from build123d import *

# Parameters (mm, degrees)
SKETCH1_R           = 22.05
BOSS_EXTRUDE1_DEPTH = 8
CUT_EXTRUDE1_REACH  = 54.573
SKETCH2_R           = 4
CUT_EXTRUDE2_REACH  = 54.573
FILLET1_SIZE        = 1
BOSS_EXTRUDE2_START = 6
SKETCH4_W           = 14
SKETCH4_H           = 20
SKETCH4_R           = 4
BOSS_EXTRUDE2_DEPTH = 6
SKETCH6_W           = 12.1
SKETCH6_H           = 8.1
CUT_EXTRUDE3_DEPTH  = 2
SKETCH7_R           = 1.25
CUT_EXTRUDE4_DEPTH  = 8
FILLET2_R           = 1


with BuildPart() as part:
    # Sketch1 → Boss-Extrude1 (new body)
    with BuildSketch(Plane.ZY):
        with Locations((25, 0)):
            Circle(SKETCH1_R)
    extrude(amount=BOSS_EXTRUDE1_DEPTH)

    # Sketch2 → Cut-Extrude1 (cut, up to next)
    with BuildSketch(Plane.ZY.offset(8), mode=Mode.PRIVATE) as cut_extrude1_sk1:
        with Locations((25, 0)):
            Circle(SKETCH2_R)
    cut_extrude1_tool1 = extrude(cut_extrude1_sk1.sketch, amount=-CUT_EXTRUDE1_REACH, mode=Mode.PRIVATE) & part.part
    add(cut_extrude1_tool1.solids().sort_by_distance((-8, 0, 25))[0], mode=Mode.SUBTRACT)

    # Sketch3 → Cut-Extrude2 (cut, up to next)
    with BuildSketch(Plane.ZY.offset(8), mode=Mode.PRIVATE) as cut_extrude2_sk1:
        with BuildLine():
            Line((12.972134752, -4.377784932), (8.743517959, -5.916875577))
            ThreePointArc((8.743517959, -5.916875577), (7.700213153, 0), (8.743517959, 5.916875577))
            Line((8.743517959, 5.916875577), (12.972134752, 4.377784932))
            ThreePointArc((12.972134752, 4.377784932), (12.200213153, 0), (12.972134752, -4.377784932))
        make_face()
    cut_extrude2_tool1 = extrude(cut_extrude2_sk1.sketch, amount=-CUT_EXTRUDE2_REACH, mode=Mode.PRIVATE) & part.part
    # Sketch3 → Cut-Extrude2 (cut, up to next)
    with BuildSketch(Plane.ZY.offset(8), mode=Mode.PRIVATE) as cut_extrude2_sk2:
        with BuildLine():
            Line((37.027865248, -4.377784932), (41.256482041, -5.916875577))
            ThreePointArc((41.256482041, -5.916875577), (42.299786847, 0), (41.256482041, 5.916875577))
            Line((41.256482041, 5.916875577), (37.027865248, 4.377784932))
            ThreePointArc((37.027865248, 4.377784932), (37.799786847, 0), (37.027865248, -4.377784932))
        make_face()
    cut_extrude2_tool2 = extrude(cut_extrude2_sk2.sketch, amount=-CUT_EXTRUDE2_REACH, mode=Mode.PRIVATE) & part.part
    add(cut_extrude2_tool1.solids().sort_by_distance((-8, 0, 10.14412))[0], mode=Mode.SUBTRACT)
    add(cut_extrude2_tool2.solids().sort_by_distance((-8, 0, 39.85588))[0], mode=Mode.SUBTRACT)

    # Fillet1
    fillet1_edges = [part.edges().sort_by_distance(p)[0] for p in [
        (0, 0, 2.95),
        (-8, 0, 2.95),
    ]]
    chamfer(fillet1_edges, length=FILLET1_SIZE)

    # Sketch4 → Boss-Extrude2 (add)
    with BuildSketch(Plane.ZY.offset(8).offset(BOSS_EXTRUDE2_START)):
        with Locations((25, -1.3)):
            Rectangle(SKETCH4_W, SKETCH4_H)
        with Locations((25, 0)):
            Circle(SKETCH4_R, mode=Mode.SUBTRACT)
    extrude(amount=-BOSS_EXTRUDE2_DEPTH)

    # Sketch6 → Cut-Extrude3 (cut)
    with BuildSketch(Plane.ZY.offset(14)):
        with Locations((25, -1.3)):
            Rectangle(SKETCH6_W, SKETCH6_H)
    extrude(amount=-CUT_EXTRUDE3_DEPTH, mode=Mode.SUBTRACT)

    # Sketch7 → Cut-Extrude4 (cut)
    with BuildSketch(Plane.ZY.offset(14)):
        with Locations((25, 5.95)):
            Circle(SKETCH7_R)
        with Locations((25, -8.55)):
            Circle(SKETCH7_R)
    extrude(amount=-CUT_EXTRUDE4_DEPTH, mode=Mode.SUBTRACT)

    # Fillet2
    fillet2_edges = [part.edges().sort_by_distance(p)[0] for p in [
        (-8, -1.3, 32),
        (-8, 8.7, 25),
        (-8, -1.3, 18),
        (-8, -11.3, 25),
    ]]
    fillet(fillet2_edges, radius=FILLET2_R)


solid = part.part
Input: part model. Units: mm. Frame: model coordinates. A direction names the side the tool comes from. Round coordinates to 2 decimals unless told otherwise and drop trailing zeros. Write each loop counter-clockwise with the first axis right and the second up, starting at its lowest first coordinate (ties: lowest second). Pieces come first, ordered by that corner, then holes.
1) Reachability of faces 4 (the flat face through (-4.056, 5.158, 39.172)), 5 (the cylindrical face through (-10.056, 7.004, 25.672)), 6 (the flat face through (-12, -11.3, 25)) from +Z, -Z, +X, -X, +Y, -Y: full face, straight path, thin tool, end or side. Return the list, or none.
2) Cut plane A-A (z = 25). Return the cut outline in (x, y).
3) Cut plane C-C (y = 0). Count the separate pieces of the cut face and the enclosed holes in it, then the cut area to 3 significant figures.
4) Draft query along Y for faces 1 (the flat face through (-12, 8.7, 25)), 2 (the flat face through (-12, -3.94, 23.57)), 3 (the flat face through (-12, -1, 32)). Return one class per face: pulls with the +Y half, pulls with the -Y half, needs draft (parallel to the pull), parting line crosses it, or undercut.
5) Cut plane B-B (x = -10). Return the cut outline in (y, z).
6) Ray query, L1, parallel to Y at x = -9.75, z = 25; L2, parallel to Y at x = -12.5, z = 20.5; L3, parallel to Z at x = -6.5, y = 2.5. Return the intervals inside material, ascending.
7) Cut plane D-D (x = -4.5). Return the cut outline in (y, z).
8) Contact query for flat-ended pins moving along their axis: P1, Ø0.8, axis at y = 6, z = 24.5, coming from the -X side; P2, Ø1, axis at x = -13, z = 20.5, coming from the -Y side; P3, Ø5, axis at x = -2, z = 21.5, coming from the +Y side. Output: stop coordinate, or through.
Geometry says:
1. face 4: +X, -X
1. face 5: -X
1. face 6: +Z, -Z, -X, -Y
2. outline: (-14, -11.3) - (-9, -11.3) arc R1 cw to (-8, -12.3) - (-8, -21.05) - (-7, -22.05) - (-1, -22.05) - (0, -21.05) - (0, -4) - (-12, -4) - (-12, -5.35) - (-14, -5.35) - (-14, -7.3) - (-6, -7.3) - (-6, -9.8) - (-14, -9.8) - close; (-14, 4) - (0, 4) - (0, 21.05) - (-1, 22.05) - (-7, 22.05) - (-8, 21.05) - (-8, 9.7) arc R1 cw to (-9, 8.7) - (-14, 8.7) - (-14, 7.2) - (-6, 7.2) - (-6, 4.7) - (-14, 4.7) - close
3. separate pieces: 4
3. enclosed holes: 0
3. area: 243 mm2
4. face 1: pulls with the +Y half
4. face 2: undercut
4. face 3: needs draft
5. outline: (-11.3, 18) - (8.7, 18) - (8.7, 32) - (-11.3, 32) - close; hole circle Ø2.5 at (-8.55, 25); hole circle Ø8 at (0, 25); hole circle Ø2.5 at (5.95, 25)
6. L1: y = -11.3 to -9.8, -7.3 to -4, 4 to 4.7, 7.2 to 8.7
6. L2: y = -11.3 to -5.35, 2.75 to 8.7
6. L3: z = 3.09 to 7.88, 12.45 to 21.88, 28.12 to 37.55, 42.12 to 46.91
7. outline: circle Ø44.1 at (0, 25); hole (-5.92, 8.74) arc R17.3 ccw to (5.92, 8.74) - (4.38, 12.97) arc R12.8 cw to (-4.38, 12.97) - close; hole (-5.92, 41.26) - (-4.38, 37.03) arc R12.8 cw to (4.38, 37.03) - (5.92, 41.26) arc R17.3 ccw to start; hole circle Ø8 at (0, 25)
8. P1: stops at x = -6
8. P2: stops at y = -11.3
8. P3: stops at y = 22.03
